Design review of the part built by this model. Coordinates are the model's own, in mm. A direction names the side the tool comes from. Coordinates: 2 decimals unless noted, no trailing zeros. Loops run counter-clockwise (first coordinate to the right, second up) from the corner with the lowest first, then second, coordinate; pieces in that order, holes last.
from build123d import *

# Parameters (mm, degrees)
SKETCH1_W           = 120
SKETCH1_H           = 80
SKETCH1_R           = 2.125
SKETCH1_R_2         = 2.5
BOSS_EXTRUDE1_DEPTH = 5
SKETCH3_W           = 15
SKETCH3_H           = 10
CUT_EXTRUDE1_DEPTH  = 5
CHAMFER2_SIZE       = 0.5
CHAMFER3_SIZE       = 0.5


with BuildPart() as part:
    # Sketch1 → Boss-Extrude1 (new body)
    with BuildSketch(Plane(origin=(0, 0, 0), x_dir=(1, 0, 0), z_dir=(0, 1, 0))):
        Rectangle(SKETCH1_W, SKETCH1_H)
        with Locations(Location((-50, 30, 0), (0, 0, 270))):
            Circle(SKETCH1_R, mode=Mode.SUBTRACT)
        with Locations(Location((-50, -30, 0), (0, 0, 90))):
            Circle(SKETCH1_R, mode=Mode.SUBTRACT)
        with Locations(Location((50, -30, 0), (0, 0, 270))):
            Circle(SKETCH1_R, mode=Mode.SUBTRACT)
        with Locations(Location((50, 30, 0), (0, 0, 90))):
            Circle(SKETCH1_R, mode=Mode.SUBTRACT)
        with Locations(Location((-26.25, 0, 0), (0, 0, 270))):
            Circle(SKETCH1_R_2, mode=Mode.SUBTRACT)
        with Locations(Location((26.25, 0, 0), (0, 0, 90))):
            Circle(SKETCH1_R_2, mode=Mode.SUBTRACT)
        with Locations(Location((-50, 0, 0), (0, 0, 270))):
            Circle(SKETCH1_R, mode=Mode.SUBTRACT)
        with Locations(Location((50, 0, 0), (0, 0, 90))):
            Circle(SKETCH1_R, mode=Mode.SUBTRACT)
        with Locations(Location((41.25, 0, 0), (0, 0, 270))):
            Circle(SKETCH1_R, mode=Mode.SUBTRACT)
        with Locations(Location((-41.25, 0, 0), (0, 0, 90))):
            Circle(SKETCH1_R, mode=Mode.SUBTRACT)
    extrude(amount=BOSS_EXTRUDE1_DEPTH)

    # Sketch3 → Cut-Extrude1 (cut)
    with BuildSketch(Plane.XZ):
        with Locations((45, -12.5)):
            Rectangle(SKETCH3_W, SKETCH3_H)
        with Locations((-45, -12.5)):
            Rectangle(SKETCH3_W, SKETCH3_H)
    extrude(amount=-CUT_EXTRUDE1_DEPTH, mode=Mode.SUBTRACT)

    # Chamfer2
    chamfer2_edges = [part.edges().sort_by_distance(p)[0] for p in [
        (-50, 5, -32.125),
        (-60, 5, 0),
        (50, 5, 27.875),
        (0, 5, 40),
        (-50, 5, 32.125),
        (50, 5, -27.875),
        (-26.25, 5, -2.5),
        (26.25, 5, 2.5),
        (-50, 5, -2.125),
        (50, 5, 2.125),
        (41.25, 5, -2.125),
        (-41.25, 5, 2.125),
        (60, 5, 0),
        (52.5, 5, -12.5),
        (45, 5, -17.5),
        (37.5, 5, -12.5),
        (45, 5, -7.5),
        (-37.5, 5, -12.5),
        (-45, 5, -17.5),
        (-52.5, 5, -12.5),
        (-45, 5, -7.5),
        (0, 5, -40),
    ]]
    chamfer(chamfer2_edges, length=CHAMFER2_SIZE)

    # Chamfer3
    chamfer3_edges = [part.edges().sort_by_distance(p)[0] for p in [
        (-50, 0, -32.125),
        (50, 0, 27.875),
        (-50, 0, 32.125),
        (50, 0, -27.875),
        (-26.25, 0, -2.5),
        (26.25, 0, 2.5),
        (-50, 0, -2.125),
        (50, 0, 2.125),
        (41.25, 0, -2.125),
        (-41.25, 0, 2.125),
        (0, 0, 40),
        (-60, 0, 0),
        (0, 0, -40),
        (60, 0, 0),
        (52.5, 0, -12.5),
        (45, 0, -7.5),
        (37.5, 0, -12.5),
        (45, 0, -17.5),
        (-37.5, 0, -12.5),
        (-45, 0, -7.5),
        (-52.5, 0, -12.5),
        (-45, 0, -17.5),
    ]]
    chamfer(chamfer3_edges, length=CHAMFER3_SIZE)


solid = part.part
Q1. The part is to be moulded in two halves that separate along Z. For faces 3 (the flat face through (-1, 5, -1)), 4 (the cylindrical face through (48.115, 2.472, 30.981)), 5 (the flat face through (-1, 2, -40)), say which applies: pulls with the +Z half, pulls with the -Z half, needs draft (parallel to the pull), parting line crosses it, or undercut.
Q2. Take a section at D-D, the plane x = 26.25. Write out the cut boundary in (y, z).
Q3. For line 1 (X direction, y = 1.5, z = 30) (3 decimals); line 2 (Z direction, x = -41.25, y = 3.65) (3 decimals); line 3 (Z direction, x = 44.5, y = 3.5), list the stretches that pass through material, from the lowest coordinate up.
Q4. Take a section at B-B, the plane z = 30. Write out the cut boundary in (x, y) (3 decimals), then the cut area to 3 significant figures.
Q5. Machinability: for faces 1 (the flat face through (60, 2, 1)), 2 (the flat face through (45, 2, -7.5)), which of the approach directions +Z, -Z, +X, -X, +Y, -Y give a long, thin tool a straight path to every point of the face, cutting with its end or side? Answer none if there is none.
Q6. Take a section at A-A, the plane y = 2.15. Give the number of separate pieces and of enclosed holes in the cut face, then the cut area to 3 significant figures.
Q7. Take a section at C-C, the plane x = -41.25. Write out the cut boundary in (y, z) (3 decimals), then the cut area to 3 significant figures.
Q8. Clearance check with flat-ended pins moving along their axes: pin 1 Ø4.5 at (x, z) = (26.25, 0) entering from -Y (1 decimal); pin 2 Ø5 at (x, z) = (50, -30) entering from +Y (3 decimals). State where each tip first meets the part, or that it passes through.
Entries:
1. face 3: needs draft
1. face 4: undercut
1. face 5: pulls with the -Z half
2. outline: (0, -39.5) - (0.5, -40) - (4.5, -40) - (5, -39.5) - (5, -3) - (4.5, -2.5) - (0.5, -2.5) - (0, -3) - close; (0, 3) - (0.5, 2.5) - (4.5, 2.5) - (5, 3) - (5, 39.5) - (4.5, 40) - (0.5, 40) - (0, 39.5) - close
3. line 1: x = -60 to -52.125, -47.875 to 47.875, 52.125 to 60
3. line 2: z = -40 to -17.5, -7.5 to -2.125, 2.125 to 40
3. line 3: z = -40 to -17.5, -7.5 to 40
4. outline: (-60, 0.5) - (-59.5, 0) - (-52.625, 0) - (-52.125, 0.5) - (-52.125, 4.5) - (-52.625, 5) - (-59.5, 5) - (-60, 4.5) - close; (-47.875, 0.5) - (-47.375, 0) - (47.375, 0) - (47.875, 0.5) - (47.875, 4.5) - (47.375, 5) - (-47.375, 5) - (-47.875, 4.5) - close; (52.125, 0.5) - (52.625, 0) - (59.5, 0) - (60, 0.5) - (60, 4.5) - (59.5, 5) - (52.625, 5) - (52.125, 4.5) - close
4. area: 556 mm2
5. face 1: +Z, -Z, +X, +Y, -Y
5. face 2: +Y, -Y
6. separate pieces: 1
6. enclosed holes: 12
6. area: 9,150 mm2
7. outline: (0, -39.5) - (0.5, -40) - (4.5, -40) - (5, -39.5) - (5, -18) - (4.5, -17.5) - (0.5, -17.5) - (0, -18) - close; (0, -7) - (0.5, -7.5) - (4.5, -7.5) - (5, -7) - (5, -2.625) - (4.5, -2.125) - (0.5, -2.125) - (0, -2.625) - close; (0, 2.625) - (0.5, 2.125) - (4.5, 2.125) - (5, 2.625) - (5, 39.5) - (4.5, 40) - (0.5, 40) - (0, 39.5) - close
7. area: 327 mm2
8. pin 1: passes through
8. pin 2: stops at y = 4.875
